The listing builds one solid part. Answer for the finished solid, in the listing's coordinates (mm). Face numbers are marked on the shaded views. A direction names the side the tool comes from. Round coordinates to 2 decimals unless told otherwise and drop trailing zeros. Order: outer loops, then holes, each group sorted by start corner. A loop starts at its lowest first (then second) coordinate and runs counter-clockwise, first axis right, second up. Notation, with made-up numbers: M -34,2 L 7,2 A30 cw 7,31 Z; hole C 50,13 d5. An arc over 180 degrees is marked long. Write item = value, one per line. Start each with the question number.
(1) A cutting plane is placed at C-C, the plane z = 4.25. Determine the outline of the cut face in (x, y), and give its area (3 significant figures).
(2) A cutting plane is placed at B-B, the plane z = 2.5. Determine the outline of the cut face in (x, y).
(3) Which of the six approach directions +Z, -Z, +X, -X, +Y, -Y give full straight-line access (tool end or side, diameter ignored) to the marked faces 4, 5 and 6?
(4) Straight lines are drawn through the part: probe 1 along Y at (x, z) = (-3.5, 7); probe 2 along Y at (x, z) = (0, 5.85); probe 3 along Z at (x, y) = (0.25, 11.75). For each, find the intervals that lie inside material, in ascending order. Write a range as from..to.
(5) A cutting plane is placed at A-A, the plane x = 0. Determine the outline of the cut face in (y, z).
(6) Each of these flat-tipped pins is pushed along its axis until it touches: pin 1 (4.5 mm diameter, centred on x = -1.5, y = 10.5, fed in from +Z); pin 2 (9 mm diameter, centred on x = 0, y = 0, fed in from -Z); pin 3 (1.5 mm diameter, centred on y = -1, z = 4, fed in from +X); pin 4 (4 mm diameter, centred on y = 11.5, z = -1, fed in from -X). Where does it stop, or does it pass through?
(7) For a pull along X with two mould halves and no side action, classify the marked faces 1, 2 and 3 as released by +X, released by -X, zero draft, split by the parting line, or undercut.
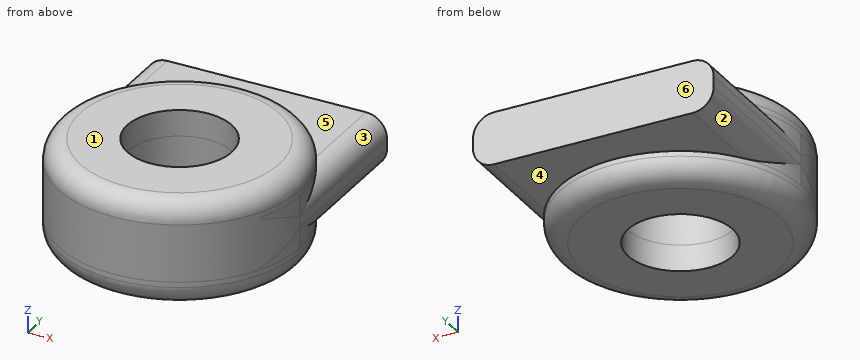
from build123d import *

# Parameters (mm, degrees)
SKETCH1_R           = 11.5
SKETCH1_R_2         = 5
SKETCH1_W           = 23
SKETCH1_H           = 4
BOSS_EXTRUDE2_DEPTH = 5
SKETCH3_R           = 11.5
BOSS_EXTRUDE3_DEPTH = 2.5
BOSS_EXTRUDE4_START = 2.5
SKETCH4_R           = 11.5
BOSS_EXTRUDE4_DEPTH = 2.5
CUT_EXTRUDE2_START  = -17.5
SKETCH5_R           = 5
CUT_EXTRUDE2_DEPTH  = 17.5
FILLET1_R           = 2


with BuildPart() as part:
    # Sketch1 → Boss-Extrude2 (new body)
    # profile 1 of 4: a face of its own
    with BuildSketch(Plane.XY):
        Circle(SKETCH1_R)
        Circle(SKETCH1_R_2, mode=Mode.SUBTRACT)
    # profile 2 of 4: a face of its own
    with BuildSketch(Plane.XY):
        with BuildLine():
            ThreePointArc((1.6e-08, 11.5), (8.131727989, 8.131727978), (11.5, 0))
            Line((11.5, 0), (11.5, 11.5))
            Line((11.5, 11.5), (1.6e-08, 11.5))
        make_face()
    # profile 3 of 4: a face of its own
    with BuildSketch(Plane.XY):
        with Locations((0, 13.5)):
            Rectangle(SKETCH1_W, SKETCH1_H)
    # profile 4 of 4: a face of its own
    with BuildSketch(Plane.XY):
        with BuildLine():
            Line((-11.5, 11.5), (-11.5, 0))
            ThreePointArc((-11.5, 0), (-8.131727978, 8.131727989), (1.6e-08, 11.5))
            Line((1.6e-08, 11.5), (-11.5, 11.5))
        make_face()
    extrude(amount=BOSS_EXTRUDE2_DEPTH)

    # Sketch3 → Boss-Extrude3 (add)
    with BuildSketch(Plane.XY.offset(5)):
        Circle(SKETCH3_R)
    extrude(amount=BOSS_EXTRUDE3_DEPTH)

    # Sketch4 → Boss-Extrude4 (add)
    with BuildSketch(Plane(origin=(0, 0, 0), x_dir=(-1, 0, 0), z_dir=(0, 0, -1)).offset(BOSS_EXTRUDE4_START)):
        Circle(SKETCH4_R)
    extrude(amount=-BOSS_EXTRUDE4_DEPTH)

    # Sketch5 → Cut-Extrude2 (cut)
    with BuildSketch(Plane.XY.offset(7.5).offset(CUT_EXTRUDE2_START)):
        with Locations(Location((0, 0, 0), (0, 0, 180))):
            Circle(SKETCH5_R)
    extrude(amount=CUT_EXTRUDE2_DEPTH, mode=Mode.SUBTRACT)

    # Fillet1
    # the kernel refuses this fillet: 2 mm, written as the material it takes off along each edge
    with BuildSketch(Plane(origin=(-11.5, 20.5, 0), x_dir=(0, 0, 1), z_dir=(0, -1, 0))) as fillet1_piece_1_section:
        with BuildLine():
            CenterArc((FILLET1_R, -FILLET1_R), FILLET1_R, 90, 90)
            Line((0, -FILLET1_R), (0, 0))
            Line((0, 0), (FILLET1_R, 0))
        make_face()
    fillet1_piece_1 = extrude(amount=25.5, mode=Mode.PRIVATE)
    fillet1_piece_1 = fillet1_piece_1 - Plane(origin=(0, 0, 0.471607453), x_dir=(1, 0, 0), z_dir=(0, 0, -1)) * Cylinder(11.5, 59, mode=Mode.PRIVATE)
    add(fillet1_piece_1, mode=Mode.SUBTRACT)
    with BuildSketch(Plane(origin=(-11.5, 20.5, 5), x_dir=(1, 0, 0), z_dir=(0, -1, 0))) as fillet1_piece_2_section:
        with BuildLine():
            CenterArc((FILLET1_R, -FILLET1_R), FILLET1_R, 90, 90)
            Line((0, -FILLET1_R), (0, 0))
            Line((0, 0), (FILLET1_R, 0))
        make_face()
    fillet1_piece_2 = extrude(amount=25.5, mode=Mode.PRIVATE)
    fillet1_piece_2 = fillet1_piece_2 - Plane(origin=(0, 0, 4.528392342), x_dir=(1, 0, 0), z_dir=(0, 0, -1)) * Cylinder(11.5, 59, mode=Mode.PRIVATE)
    add(fillet1_piece_2, mode=Mode.SUBTRACT)
    with BuildSketch(Plane(origin=(11.5, -5, 0), x_dir=(0, 0, 1), z_dir=(0, 1, 0))) as fillet1_piece_3_section:
        with BuildLine():
            CenterArc((FILLET1_R, -FILLET1_R), FILLET1_R, 90, 90)
            Line((0, -FILLET1_R), (0, 0))
            Line((0, 0), (FILLET1_R, 0))
        make_face()
    fillet1_piece_3 = extrude(amount=25.5, mode=Mode.PRIVATE)
    fillet1_piece_3 = fillet1_piece_3 - Plane(origin=(0, 0, 0.471608914), x_dir=(1, 0, 0), z_dir=(0, 0, -1)) * Cylinder(11.5, 59, mode=Mode.PRIVATE)
    add(fillet1_piece_3, mode=Mode.SUBTRACT)
    with BuildSketch(Plane(origin=(11.5, 20.5, 5), x_dir=(0, 0, -1), z_dir=(0, -1, 0))) as fillet1_piece_4_section:
        with BuildLine():
            CenterArc((FILLET1_R, -FILLET1_R), FILLET1_R, 90, 90)
            Line((0, -FILLET1_R), (0, 0))
            Line((0, 0), (FILLET1_R, 0))
        make_face()
    fillet1_piece_4 = extrude(amount=25.5, mode=Mode.PRIVATE)
    fillet1_piece_4 = fillet1_piece_4 - Plane(origin=(0, 0, 4.528391109), x_dir=(1, 0, 0), z_dir=(0, 0, -1)) * Cylinder(11.5, 59, mode=Mode.PRIVATE)
    add(fillet1_piece_4, mode=Mode.SUBTRACT)
    with BuildSketch(Plane(origin=(0, 0, 7.5), x_dir=(1, 0, 0), z_dir=(0, -1, 0))) as fillet1_piece_5:
        with BuildLine():
            CenterArc((11.5 - FILLET1_R, -FILLET1_R), FILLET1_R, 0, 90)
            Line((11.5 - FILLET1_R, 0), (11.5, 0))
            Line((11.5, 0), (11.5, -FILLET1_R))
        make_face()
    revolve(axis=Axis((0, 0, 7.5), (0, 0, 1)), mode=Mode.SUBTRACT)
    with BuildSketch(Plane(origin=(0, 0, -2.5), x_dir=(-1, 0, 0), z_dir=(0, -1, 0))) as fillet1_piece_6:
        with BuildLine():
            CenterArc((11.5 - FILLET1_R, -FILLET1_R), FILLET1_R, 0, 90)
            Line((11.5 - FILLET1_R, 0), (11.5, 0))
            Line((11.5, 0), (11.5, -FILLET1_R))
        make_face()
    revolve(axis=Axis((0, 0, -2.5), (0, 0, -1)), mode=Mode.SUBTRACT)


solid = part.part
Reported:
q1.outline = M -11.06,3.15 A11.5 ccw long 11.06,3.15 L 11.06,15.5 L -11.06,15.5 Z; hole C 0,0 d10
q1.area = 474 mm²
q2.outline = M -11.5,0 A11.5 ccw 11.5,0 L 11.5,15.5 L -11.5,15.5 Z; hole C 0,0 d10
q3.face_4 = -Z, +Y
q3.face_5 = +Z, +Y
q3.face_6 = +Z, -Z, +X, -X, +Y
q4.probe_1 = -10.24..-3.57, 3.57..10.24
q4.probe_2 = -11.47..-5, 5..11.47
q4.probe_3 = 0..5
q5.outline = M -11.5,-0.5 A2 ccw -9.5,-2.5 L -5,-2.5 L -5,7.5 L -9.5,7.5 A2 ccw -11.5,5.5 Z; M 5,-2.5 L 9.5,-2.5 A2 ccw 11.5,-0.5 L 11.5,0 L 15.5,0 L 15.5,5 L 11.5,5 L 11.5,5.5 A2 ccw 9.5,7.5 L 5,7.5 Z
q6.pin_1 = 7.5
q6.pin_2 = through
q6.pin_3 = 11.5
q6.pin_4 = -11.23
q7.face_1 = zero draft
q7.face_2 = released by -X
q7.face_3 = released by +X
